from build123d import *

# Parameters (mm, degrees)
SKETCH_1_R      = 2.1
EXTRUDE_1_DEPTH = 10
EXTRUDE_2_DEPTH = 90
SKETCH_3_R      = 2.1
EXTRUDE_3_DEPTH = 10
EXTRUDE_4_DEPTH = 90
EXTRUDE_5_DEPTH = 5
SKETCH_6_R      = 2.1
EXTRUDE_6_DEPTH = 10


with BuildPart() as part:
    # Sketch 1 → Extrude 1 (new body)
    with BuildSketch(Plane(origin=(0, 139.195974268, 0), x_dir=(1, 0, 0), z_dir=(0, 1, 0))):
        Polygon((108.058980694, -32.273129836), (128.058980694, -32.273129836), (128.058980694, -68.273129836), (123.058980694, -68.273129836), (123.058980694, -56.273129836), (108.058980694, -56.273129836), align=None)
        with Locations(Location((120.058980694, -40.273129836, 0), (0, 0, 180))):
            Circle(SKETCH_1_R, mode=Mode.SUBTRACT)
    extrude(amount=EXTRUDE_1_DEPTH)

    # Sketch 2 → Extrude 2 (add)
    with BuildSketch(Plane(origin=(0, 149.195974268, 0), x_dir=(1, 0, 0), z_dir=(0, 1, 0))):
        Polygon((128.058980694, -32.273129836), (125.058980694, -32.273129836), (125.058980694, -48.273129836), (108.058980694, -48.273129836), (108.058980694, -56.273129836), (123.058980694, -56.273129836), (123.058980694, -68.273129836), (128.058980694, -68.273129836), align=None)
    extrude(amount=EXTRUDE_2_DEPTH)



with BuildPart() as body_2:
    # Sketch 3 → Extrude 3 (new body)
    with BuildSketch(Plane(origin=(0, 139.195974268, 0), x_dir=(1, 0, 0), z_dir=(0, 1, 0))):
        Polygon((123.058980694, -110.773129836), (123.058980694, -122.773129836), (108.058980694, -122.773129836), (108.058980694, -146.773129836), (128.058980694, -146.773129836), (128.058980694, -110.773129836), align=None)
        with Locations(Location((120.058980694, -138.773129836, 0), (0, 0, 180))):
            Circle(SKETCH_3_R, mode=Mode.SUBTRACT)
    extrude(amount=EXTRUDE_3_DEPTH)

    # Sketch 4 → Extrude 4 (add)
    with BuildSketch(Plane(origin=(0, 149.195974268, 0), x_dir=(1, 0, 0), z_dir=(0, 1, 0))):
        Polygon((123.058980694, -110.773129836), (123.058980694, -122.773129836), (108.058980694, -122.773129836), (108.058980694, -130.773129836), (125.058980694, -130.773129836), (125.058980694, -146.773129836), (128.058980694, -146.773129836), (128.058980694, -110.773129836), align=None)
    extrude(amount=EXTRUDE_4_DEPTH)


with BuildPart() as part_1:
    add(part.part)

    add(body_2.part)  # Extrude 5 merges body 2
    # Sketch 5 → Extrude 5 (add)
    with BuildSketch(Plane(origin=(128.058980694, 0, 0), x_dir=(0, 0, -1), z_dir=(1, 0, 0))):
        Polygon((-68.273129836, 224.145974268), (-68.273129836, 209.145974268), (-82.439796503, 194.145974268), (-68.273129836, 179.145974268), (-68.273129836, 164.145974268), (-89.523129836, 186.645974268), (-110.773129836, 164.145974268), (-110.773129836, 179.145974268), (-96.60646317, 194.145974268), (-110.773129836, 209.145974268), (-110.773129836, 224.145974268), (-89.523129836, 201.645974268), align=None)
    extrude(amount=-EXTRUDE_5_DEPTH)

    # Sketch 6 → Extrude 6 (add)
    with BuildSketch(Plane(origin=(0, 239.195974268, 0), x_dir=(1, 0, 0), z_dir=(0, 1, 0))):
        Polygon((108.058980694, -56.273129836), (108.058980694, -32.273129836), (128.058980694, -32.273129836), (128.058980694, -146.773129836), (108.058980694, -146.773129836), (108.058980694, -122.773129836), (123.058980694, -122.773129836), (123.058980694, -56.273129836), align=None)
        with Locations(Location((118.058980694, -40.273129836, 0), (0, 0, 180))):
            Circle(SKETCH_6_R, mode=Mode.SUBTRACT)
        with Locations(Location((118.058980694, -138.773129836, 0), (0, 0, 180))):
            Circle(SKETCH_6_R, mode=Mode.SUBTRACT)
    extrude(amount=EXTRUDE_6_DEPTH)


solid = part_1.part
Source: CAD feature listing. Evaluate the final solid. Frame: model axes, mm. A direction names the side the tool comes from. Coordinates: 2 decimals unless noted, no trailing zeros. Loops run counter-clockwise (first coordinate to the right, second up) from the corner with the lowest first, then second, coordinate; pieces in that order, holes last. Notation, with made-up numbers: (51, -11.5) - (71, -11.5) arc R20 ccw to (71, 13.5) - close; hole circle Ø3 at (12, 44). An arc over 180 degrees is marked (long way). One line per item, written item: value. Start each with the question number.
1. Section D-D (z = 86.5). Return the cut outline in (x, y), and give its area (3 significant figures).
2. Mould query, pull axis Z, two halves, no side actions, for faces 1 (the flat face through (126, 194, 68.273)), 2 (the flat face through (128.059, 193, 89)), 3 (the flat face through (126, 194, 146.773)). Classes: pulls with the +Z half, pulls with the -Z half, needs draft (parallel to the pull), parting line crosses it, or undercut.
3. Contact query for flat-ended pins moving along their axis: P1, Ø4.5, axis at x = 118.5, y = 171.5, coming from the +Z side; P2, Ø3.5, axis at x = 120.06, z = 40.27, coming from the -Y side; P3, Ø13, axis at y = 189.5, z = 42, coming from the -X side; P4, Ø6, axis at x = 116.5, y = 228, coming from the -Z side. Output: stop coordinate, or through.
4. Section A-A (x = 111). Return the cut outline in (y, z), and give its area (3 significant figures).
5. Ray query, L1, parallel to Z at x = 115.5, y = 214; L2, parallel to Z at x = 126.5, y = 219; L3, parallel to X at y = 171, z = 140.5. Return the intervals inside material, ascending.
6. Section B-B (y = 166). Return the cut outline in (x, z).
7. Section C-C (y = 196.5). Return the cut outline in (x, z).
8. Set-up query: faces 4 (the flat face through (126, 151, 110.773)), 5 (the flat face through (126, 194, 110.773)), 6 (the flat face through (116.7, 239.196, 136.9)), 7 (the flat face through (117, 149.196, 40)). Return all of +Z, -Z, +X, -X, +Y, -Y with unobstructed straight access to the full face (end or side cutting, diameter ignored); none if empty.
Verdict:
1. outline: (123.06, 183.45) - (128.06, 183.45) - (128.06, 204.85) - (123.06, 204.85) - close; (123.06, 239.2) - (128.06, 239.2) - (128.06, 249.2) - (123.06, 249.2) - close
1. area: 157 mm2
2. face 1: undercut
2. face 2: needs draft
2. face 3: pulls with the +Z half
3. P1: stops at z = 130.77
3. P2: stops at y = 239.2
3. P3: stops at x = 108.06
3. P4: stops at z = 48.27
4. outline: (139.2, 32.27) - (149.2, 32.27) - (149.2, 48.27) - (239.2, 48.27) - (239.2, 32.27) - (249.2, 32.27) - (249.2, 56.27) - (139.2, 56.27) - close; (139.2, 122.77) - (249.2, 122.77) - (249.2, 146.77) - (239.2, 146.77) - (239.2, 130.77) - (149.2, 130.77) - (149.2, 146.77) - (139.2, 146.77) - close
4. area: 2,400 mm2
5. L1: z = 48.27 to 56.27, 122.77 to 130.77
5. L2: z = 32.27 to 73.13, 105.91 to 146.77
5. L3: x = 125.06 to 128.06
6. outline: (108.06, 48.27) - (125.06, 48.27) - (125.06, 32.27) - (128.06, 32.27) - (128.06, 70.02) - (123.06, 70.02) - (123.06, 56.27) - (108.06, 56.27) - close; (108.06, 122.77) - (123.06, 122.77) - (123.06, 109.02) - (128.06, 109.02) - (128.06, 146.77) - (125.06, 146.77) - (125.06, 130.77) - (108.06, 130.77) - close
7. outline: (108.06, 48.27) - (125.06, 48.27) - (125.06, 32.27) - (128.06, 32.27) - (128.06, 68.27) - (123.06, 68.27) - (123.06, 56.27) - (108.06, 56.27) - close; (108.06, 122.77) - (123.06, 122.77) - (123.06, 110.77) - (128.06, 110.77) - (128.06, 146.77) - (125.06, 146.77) - (125.06, 130.77) - (108.06, 130.77) - close; (123.06, 80.22) - (128.06, 80.22) - (128.06, 98.83) - (123.06, 98.83) - close
8. face 4: +X, -X, -Y
8. face 5: +X, -X
8. face 6: +Z, -X
8. face 7: -Z, -X
